Geometry check sheet. Reference: the model listing, model coordinates, mm. A direction names the side the tool comes from. Round coordinates to 2 decimals unless told otherwise and drop trailing zeros. Order: outer loops, then holes, each group sorted by start corner. A loop starts at its lowest first (then second) coordinate and runs counter-clockwise, first axis right, second up.
(1) Cross-section at C-C on y = 81.5. Enter the section's corners in (x, z).
(2) Cross-section at D-D on x = 27. Enter the section's corners in (y, z), and give its area (3 significant figures).
(3) Draft check along Y on faces 1 (the face through (60, 129, -300)), 2 (the face through (59, 0, -4)), 3 (the face through (25.256, 228.466, -4.2)). Enter one of: pulls with the +Y half, pulls with the -Y half, needs draft (parallel to the pull), parting line crosses it, or undercut.
(4) Gauge pin test, flat ends, axial feed: P1, Ø8, axis at y = 48, z = 17, coming from the -X side; P2, Ø4, axis at x = 39, z = 122.5, coming from the -Y side. Record the tip position at first contact, or that the pin passes through.
(5) Set-up check for faces 4 (the face through (60, 129, 300)), 5 (the face through (25.83, 11.63, -4.2)), 6 (the face through (66.67, 220.83, -4.2)): record each of +Z, -Z, +X, -X, +Y, -Y from which the full face is reachable in a straight line by a thin tool's end or side.
(6) Cross-section at A-A on x = 94. Enter the section's corners in (y, z), and give its area (3 significant figures).
(7) Thickness scan on L1, parallel to X at y = 49, z = 43; L2, parallel to Y at x = 42, z = -127.5; L3, parallel to Y at x = 10.5, z = -222. Record the ranges inside material, lowest first.
(8) Cross-section at B-B on z = 14. Enter the section's corners in (x, y), and give its area (3 significant figures).
from build123d import *

# Parameters (mm, degrees)
BASESBEAM_START = -300
BASESBEAM_DEPTH = 600
TOEFILLET_R     = 6


# Read off the part's stored shape, not the designer's step: BaseSbeam
with BuildPart() as part:
    # BaseSbeam outline → BaseSbeam (new body)
    with BuildSketch(Plane.XY.offset(BASESBEAM_START)):
        with BuildLine():
            Line((0, 7.324658955), (0, 0))
            Line((0, 0), (120, 0))
            Line((120, 0), (120, 7.324658955))
            Line((120, 7.324658955), (73.927072128, 15.004040437))
            ThreePointArc((73.927072128, 15.004040437), (66.743714332, 19.084299589), (63.9, 26.840744185))
            Line((63.9, 26.840744185), (63.9, 213.159255815))
            ThreePointArc((63.9, 213.159255815), (66.743714332, 220.915700411), (73.927072128, 224.995959563))
            Line((73.927072128, 224.995959563), (120, 232.675341045))
            Line((120, 232.675341045), (120, 240))
            Line((120, 240), (0, 240))
            Line((0, 240), (0, 232.675341045))
            Line((0, 232.675341045), (46.072927872, 224.995959563))
            ThreePointArc((46.072927872, 224.995959563), (53.256285668, 220.915700411), (56.1, 213.159255815))
            Line((56.1, 213.159255815), (56.1, 26.840744185))
            ThreePointArc((56.1, 26.840744185), (53.256285668, 19.084299589), (46.072927872, 15.004040437))
            Line((46.072927872, 15.004040437), (0, 7.324658955))
        make_face()
    extrude(amount=BASESBEAM_DEPTH)

    # ToeFillet
    toefillet_edges = [part.edges().sort_by_distance(p)[0] for p in [
        (120, 7.324658955, 0),
        (120, 232.675341045, 0),
        (0, 232.675341045, 0),
        (0, 7.324658955, 0),
    ]]
    fillet(toefillet_edges, radius=TOEFILLET_R)


solid = part.part
Found:
1. outline: (56.1, -300) - (63.9, -300) - (63.9, 300) - (56.1, 300) - close
2. outline: (0, -300) - (11.82, -300) - (11.82, 300) - (0, 300) - close; (228.18, -300) - (240, -300) - (240, 300) - (228.18, 300) - close
2. area: 14,200 mm2
3. face 1: needs draft
3. face 2: pulls with the -Y half
3. face 3: undercut
4. P1: stops at x = 56.1
4. P2: stops at y = 0
5. face 4: +Z, +X, -X, +Y, -Y
5. face 5: +Z, -Z, -X
5. face 6: +Z, -Z, +X
6. outline: (0, -300) - (11.66, -300) - (11.66, 300) - (0, 300) - close; (228.34, -300) - (240, -300) - (240, 300) - (228.34, 300) - close
6. area: 14,000 mm2
7. L1: x = 56.1 to 63.9
7. L2: y = 0 to 14.33, 225.67 to 240
7. L3: y = 0 to 9.07, 230.93 to 240
8. outline: (0, 0) - (120, 0) - (120, 2.24) arc R6 ccw to (114.99, 8.16) - (73.93, 15) arc R12 cw to (63.9, 26.84) - (63.9, 213.16) arc R12 cw to (73.93, 225) - (114.99, 231.84) arc R6 ccw to (120, 237.76) - (120, 240) - (0, 240) - (0, 237.76) arc R6 ccw to (5.01, 231.84) - (46.07, 225) arc R12 cw to (56.1, 213.16) - (56.1, 26.84) arc R12 cw to (46.07, 15) - (5.01, 8.16) arc R6 ccw to (0, 2.24) - close
8. area: 4,630 mm2
